CAD build for the part. Positions are in the model's coordinates, mm. A direction names the side the tool comes from. Round coordinates to 2 decimals unless told otherwise and drop trailing zeros. Order: outer loops, then holes, each group sorted by start corner. A loop starts at its lowest first (then second) coordinate and runs counter-clockwise, first axis right, second up. Notation, with made-up numbers: M 33,-39.75 L 59,-39.75 A27 cw 59,-7.75 Z; hole C 3.25,28 d8. An arc over 180 degrees is marked long. Put each result on its own line as item: value.
```python
from build123d import *

# Parameters (mm, degrees)
PAD_DEPTH              = 17.15
POCKET_DEPTH           = 15.51
FILLET_R               = 1.5
SKETCH002_R            = 3
HOLE_DEPTH             = 25
LINEARPATTERN_COUNT    = 7
LINEARPATTERN_PITCH    = 10.041667
SKETCH003_R            = 3
HOLE001_DEPTH          = 25
LINEARPATTERN001_COUNT = 7
LINEARPATTERN001_PITCH = 10.041667
PAD001_DEPTH           = 2.41
SKETCH005_R            = 2.38
PAD002_DEPTH           = 2.41
SKETCH006_R            = 1.5
POCKET001_DEPTH        = 223.463007
REVOLUTION_ANGLE       = 90


with BuildPart() as part:
    # Sketch → Pad (new body)
    with BuildSketch(Plane.XY):
        with BuildLine():
            Line((-30.905, 18.795), (30.905, 18.795))
            ThreePointArc((39.905, 9.795), (37.268961, 16.158961), (30.905, 18.795))
            Line((39.905, 9.795), (39.905, -9.795))
            ThreePointArc((30.905, -18.795), (37.268961, -16.158961), (39.905, -9.795))
            Line((30.905, -18.795), (-30.905, -18.795))
            ThreePointArc((-39.905, -9.795), (-37.268961, -16.158961), (-30.905, -18.795))
            Line((-39.905, -9.795), (-39.905, 9.795))
            ThreePointArc((-30.905, 18.795), (-37.268961, 16.158961), (-39.905, 9.795))
        make_face()
    extrude(amount=PAD_DEPTH)

    # Sketch001 (on Face9 of Pad) → Pocket (cut)
    with BuildSketch(Plane(origin=(0, 0, 0), x_dir=(1, 0, 0), z_dir=(0, 0, -1))):
        with BuildLine():
            Line((-30.395, 18.29), (30.395, 18.29))
            ThreePointArc((39.395, 9.29), (36.758961, 15.653961), (30.395, 18.29))
            Line((39.395, 9.29), (39.395, -9.29))
            ThreePointArc((30.395, -18.29), (36.758961, -15.653961), (39.395, -9.29))
            Line((30.395, -18.29), (-30.395, -18.29))
            ThreePointArc((-39.395, -9.29), (-36.758961, -15.653961), (-30.395, -18.29))
            Line((-39.395, -9.29), (-39.395, 9.29))
            ThreePointArc((-30.395, 18.29), (-36.758961, 15.653961), (-39.395, 9.29))
        make_face()
    extrude(amount=-POCKET_DEPTH, mode=Mode.SUBTRACT)

    # Fillet
    fillet_edges = [part.edges().sort_by_distance(p)[0] for p in [
        (-39.905, 0, 17.15),
        (-37.268961, 16.158961, 17.15),
        (0, 18.795, 17.15),
        (37.268961, 16.158961, 17.15),
        (39.905, 0, 17.15),
        (37.268961, -16.158961, 17.15),
        (0, -18.795, 17.15),
        (-37.268961, -16.158961, 17.15),
    ]]
    fillet(fillet_edges, radius=FILLET_R)

    # Sketch002 (on Face8 of Fillet) → Hole (cut)
    with BuildSketch(Plane.XY.offset(17.15)):
        with Locations((-30.155, 8.7875)):
            Circle(SKETCH002_R)
    hole = extrude(amount=-HOLE_DEPTH, mode=Mode.SUBTRACT)

    # LinearPattern: Hole ×7
    with Locations(*[(i * LINEARPATTERN_PITCH, 0, 0) for i in range(1, LINEARPATTERN_COUNT)]):
        add(hole, mode=Mode.SUBTRACT)

    # Sketch003 (on Face8 of LinearPattern) → Hole001 (cut)
    with BuildSketch(Plane.XY.offset(17.15)):
        with Locations((-30.155, -8.7875)):
            Circle(SKETCH003_R)
    hole001 = extrude(amount=-HOLE001_DEPTH, mode=Mode.SUBTRACT)

    # LinearPattern001: Hole001 ×7
    with Locations(*[(i * LINEARPATTERN001_PITCH, 0, 0) for i in range(1, LINEARPATTERN001_COUNT)]):
        add(hole001, mode=Mode.SUBTRACT)

    # Sketch004 → Pad001 (join)
    with BuildSketch(Plane.XY):
        Polygon((39.905, 6.605), (39.905, -6.605), (46.288485, -1.918481), (46.28848, 1.918485), align=None)
    pad001 = extrude(amount=PAD001_DEPTH)

    # Mirrored: Pad001 across Sketch004 V_Axis
    add(pad001.mirror(Plane(origin=(0, 0, 0), x_dir=(0, 0, 1), z_dir=(1, 0, 0))))

    # Sketch005 → Pad002 (join)
    with BuildSketch(Plane.XY):
        with Locations((-44.88, 0)):
            Circle(SKETCH005_R)
    pad002 = extrude(amount=PAD002_DEPTH)

    # Mirrored001: Pad002 across Sketch005 V_Axis
    add(pad002.mirror(Plane(origin=(0, 0, 0), x_dir=(0, 0, 1), z_dir=(1, 0, 0))))

    # Sketch006 → Pocket001 (cut, through all)
    with BuildSketch(Plane.XY):
        with Locations((-44.875, 0)):
            Circle(SKETCH006_R)
    pocket001 = extrude(amount=POCKET001_DEPTH, mode=Mode.SUBTRACT)

    # Mirrored002: Pocket001 across Sketch006 V_Axis
    add(pocket001.mirror(Plane(origin=(0, 0, 0), x_dir=(0, 0, 1), z_dir=(1, 0, 0))), mode=Mode.SUBTRACT)

    # Sketch007 (on Face5 of Mirrored002) → Revolution (revolve)
    with BuildSketch(Plane.XY.offset(2.41)):
        with BuildLine():
            Line((-39.905, 1.699299), (-39.905, 0))
            Line((-39.905, 0), (-40.863067, 0))
            ThreePointArc((-39.905, 1.699299), (-40.601365, 0.972181), (-40.863067, 0))
        make_face()
    revolution = revolve(axis=Axis((0, 0, 0), (1, 0, 0)), revolution_arc=REVOLUTION_ANGLE)

    # Mirrored003: Revolution across Sketch007 V_Axis
    add(revolution.mirror(Plane(origin=(0, 0, 2.41), x_dir=(0, 0, 1), z_dir=(1, 0, 0))))


solid = part.part
```
Item 1: Band-saw the part on D-D on x = -22. Give the cut face in (y, z) (3 decimals).
Answers below:
outline: M -18.795,0 L -18.29,0 L -18.29,15.51 L -11.12,15.51 L -11.12,17.15 L -17.295,17.15 A1.5 ccw -18.795,15.65 Z; M -6.455,15.51 L 6.455,15.51 L 6.455,17.15 L -6.455,17.15 Z; M 11.12,15.51 L 18.29,15.51 L 18.29,0 L 18.795,0 L 18.795,15.65 A1.5 ccw 17.295,17.15 L 11.12,17.15 Z
Item 2: Pin check, flat tips, straight feed: P1, Ø10, axis at y = -3.5, z = 13, coming from the +X side (3 decimals); P2, Ø9.5, axis at x = -20.11, y = -8.79, coming from the +Z side; P3, Ø8, axis at x = 30.1, y = -8.79, coming from the -Z side; P4, Ø5, axis at x = 20.05, y = 8.79, coming from the +Z side. Stop position of each tip, or through.
Answers below:
P1: x = 39.905
P2: z = 17.15
P3: z = 15.51
P4: through
Item 3: Tool access for faces 1 (the cylindrical face through (-0.421, -5.813, 16.341)), 2 (the cylindrical face through (36.83, -15.58, 7.65)): list every direction of +Z, -Z, +X, -X, +Y, -Y with a clear straight run to the whole face (end or side of a thin tool).
Answers below:
face 1: +Z, -Z
face 2: -Z
Item 4: Mould opens along Y. For faces 3 (the flat face through (43.052, -4.295, 1.188)), 4 (the flat face through (43, 0, 2.41)), 5 (the cylindrical face through (-27.294, -7.886, 16.341)) say: pulls with the +Y half, pulls with the -Y half, needs draft (parallel to the pull), parting line crosses it, or undercut.
Answers below:
face 3: pulls with the -Y half
face 4: needs draft
face 5: undercut
Item 5: Band-saw the part on A-A on x = -0.03. State how many separate pieces and enclosed holes the cut face has, and give its area (3 significant figures).
Answers below:
separate pieces: 3
enclosed holes: 0
area: 56.7 mm²
Item 6: Probe line 1 along Y through (x, z) = (10.5, 14.5) (3 decimals); line 2 along X through (y, z) = (-4, 9.5) (3 decimals); line 3 along Z through (x, y) = (15, 5.5). List the from-to ranges inside material, lowest first. Write a range as [from, to].
Answers below:
line 1: [-18.795, -18.29], [18.29, 18.795]
line 2: [-39.905, -39.395], [39.395, 39.905]
line 3: [15.51, 17.15]
Item 7: Band-saw the part on B-B on z = 13.25. Give the cut face in (x, y) (3 decimals).
Answers below:
outline: M -39.905,-9.795 A9 ccw -30.905,-18.795 L 30.905,-18.795 A9 ccw 39.905,-9.795 L 39.905,9.795 A9 ccw 30.905,18.795 L -30.905,18.795 A9 ccw -39.905,9.795 Z; hole M -39.395,-9.29 A9 ccw -30.395,-18.29 L 30.395,-18.29 A9 ccw 39.395,-9.29 L 39.395,9.29 A9 ccw 30.395,18.29 L -30.395,18.29 A9 ccw -39.395,9.29 Z
